from build123d import *

# Parameters (mm, degrees)
SKETCH1_W                = 114.3
SKETCH1_H                = 101.6
BOSS_EXTRUDE1_DEPTH      = 3.175
SKETCH2_W                = 114.3
SKETCH2_H                = 25.4
SKETCH2_H_2              = 19.05
BOSS_EXTRUDE2_DEPTH      = 3.175
M3_CLEARANCE_HOLE1_D     = 3.4
M3_CLEARANCE_HOLE1_DEPTH = 6.35
M3_CLEARANCE_HOLE1_TIP   = 1.021463052


with BuildPart() as part:
    # Sketch1 → Boss-Extrude1 (new body)
    with BuildSketch(Plane(origin=(0, 0, 0), x_dir=(1, 0, 0), z_dir=(0, 1, 0))):
        Rectangle(SKETCH1_W, SKETCH1_H)
    extrude(amount=BOSS_EXTRUDE1_DEPTH)

    # Sketch2 → Boss-Extrude2 (add)
    # profile 1 of 4: a face of its own
    with BuildSketch(Plane(origin=(0, 3.175, 0), x_dir=(1, 0, 0), z_dir=(0, 1, 0))):
        with BuildLine():
            Line((-76.2, -50.8), (-57.15, -50.8))
            Line((-57.15, -50.8), (-57.15, 50.8))
            Line((-57.15, 50.8), (-76.2, 50.8))
            Line((-76.2, 50.8), (-76.2, -25.4))
            ThreePointArc((-76.2, -25.4), (-88.9, -38.1), (-76.2, -50.8))
        make_face()
        with BuildLine():
            ThreePointArc((-76.2, -34.1), (-72.2, -38.1), (-76.2, -42.1))
            ThreePointArc((-76.2, -42.1), (-80.2, -38.1), (-76.2, -34.1))
        make_face(mode=Mode.SUBTRACT)
    # profile 2 of 4: a face of its own
    with BuildSketch(Plane(origin=(0, 3.175, 0), x_dir=(1, 0, 0), z_dir=(0, 1, 0))):
        with Locations((0, -63.5)):
            Rectangle(SKETCH2_W, SKETCH2_H)
    # profile 3 of 4: a face of its own
    with BuildSketch(Plane(origin=(0, 3.175, 0), x_dir=(1, 0, 0), z_dir=(0, 1, 0))):
        with BuildLine():
            Line((57.15, -50.8), (76.2, -50.8))
            ThreePointArc((76.2, -50.8), (88.9, -38.1), (76.2, -25.4))
            Line((76.2, -25.4), (76.2, 50.8))
            Line((76.2, 50.8), (57.15, 50.8))
            Line((57.15, 50.8), (57.15, -50.8))
        make_face()
        with BuildLine():
            ThreePointArc((76.2, -42.1), (72.2, -38.1), (76.2, -34.1))
            ThreePointArc((76.2, -34.1), (80.2, -38.1), (76.2, -42.1))
        make_face(mode=Mode.SUBTRACT)
    # profile 4 of 4: a face of its own
    with BuildSketch(Plane(origin=(0, 3.175, 0), x_dir=(1, 0, 0), z_dir=(0, 1, 0))):
        with Locations((0, 60.325)):
            Rectangle(SKETCH2_W, SKETCH2_H_2)
    extrude(amount=-BOSS_EXTRUDE2_DEPTH)

    # M3 Clearance Hole1
    with Locations(Plane(origin=(0, 3.175, 0), x_dir=(1, 0, 0), z_dir=(0, 1, 0))):
        with Locations((-76.2, -29.6), (-76.2, -46.6), (76.2, -29.6), (76.2, -46.6)):
            Hole(M3_CLEARANCE_HOLE1_D / 2, depth=M3_CLEARANCE_HOLE1_DEPTH)
            with Locations((0, 0, -(M3_CLEARANCE_HOLE1_DEPTH + M3_CLEARANCE_HOLE1_TIP / 2))):  # 118° drill point
                Cone(0, M3_CLEARANCE_HOLE1_D / 2, M3_CLEARANCE_HOLE1_TIP, mode=Mode.SUBTRACT)


solid = part.part
Check sheet for the modelled part. Datum: model origin and axes. Units: mm. Give positions to 0.01 mm unless a question says otherwise; leave off trailing zeros. Loops run counter-clockwise (first coordinate to the right, second up) from the corner with the lowest first, then second, coordinate; pieces in that order, holes last. Notation, with made-up numbers: M 24.5,3 L 28.5,3 A28 cw 28.5,34 Z; hole C 5.5,45.5 d9. An arc over 180 degrees is marked long. Return JSON: item names as keys, results as strings. Group by question number.
1. Go/stop test with flat-tipped pins: pin 1 (1.6 mm diameter, centred on y = 1.5, z = -12.5, fed in from -X); pin 2 (1 mm diameter, centred on x = 69.5, y = 2, fed in from +Z); pin 3 (1.5 mm diameter, centred on y = 2.5, z = -24.5, fed in from +X). Record where each tip stops, or that it passes through.
2. Thickness scan on L1, parallel to X at y = 1.05, z = 38.1; L2, parallel to X at y = 3, z = 35; L3, parallel to X at y = 2.15, z = 52. Record the ranges inside material, lowest first.
3. Cross-section at A-A on z = 38.1. Record the boundary of the cut face in (x, y) (3 decimals).
4. Cross-section at B-B on y = 0.6. Record the boundary of the cut face in (x, z).
5. Cross-section at D-D on z = 56.5. Record the boundary of the cut face in (x, y) (3 decimals).
6. Mould release check, pull along Z, two halves, no side actions. Record for faces 1 (the cylindrical face through (-88.897, 1.61, 37.821)), 2 (the cylindrical face through (-73.8, 1.6, 34.9)), 3 (the flat face through (-1, 3.175, 2)), 4 (the cylindrical face through (72.651, 1.61, 36.254)): released by +Z, released by -Z, zero draft, split by the parting line, or undercut.
7. Cross-section at C-C on z = -19.5. Record the boundary of the cut face in (x, y) (3 decimals).
Return value:
{
 "1": {"pin 1": "x = -76.2", "pin 2": "z = 50.8", "pin 3": "x = 76.2"},
 "2": {"L1": "-88.9 to -80.2, -72.2 to 72.2, 80.2 to 88.9", "L2": "-88.52 to -78.73, -73.67 to 73.67, 78.73 to 88.52", "L3": "-57.15 to 57.15"},
 "3": {"outline": "M -88.9,0 L -80.2,0 L -80.2,3.175 L -88.9,3.175 Z; M -72.2,0 L 72.2,0 L 72.2,3.175 L -72.2,3.175 Z; M 80.2,0 L 88.9,0 L 88.9,3.175 L 80.2,3.175 Z"},
 "4": {"outline": "M -76.2,-50.8 L -57.15,-50.8 L -57.15,-69.85 L 57.15,-69.85 L 57.15,-50.8 L 76.2,-50.8 L 76.2,25.4 A12.7 ccw 76.2,50.8 L 57.15,50.8 L 57.15,76.2 L -57.15,76.2 L -57.15,50.8 L -76.2,50.8 A12.7 ccw -76.2,25.4 Z; hole C -76.2,38.1 d8; hole C -76.2,29.6 d3.4; hole C -76.2,46.6 d3.4; hole C 76.2,38.1 d8; hole C 76.2,29.6 d3.4; hole C 76.2,46.6 d3.4"},
 "5": {"outline": "M -57.15,0 L 57.15,0 L 57.15,3.175 L -57.15,3.175 Z"},
 "6": {"face 1": "split by the parting line", "face 2": "undercut", "face 3": "zero draft", "face 4": "undercut"},
 "7": {"outline": "M -76.2,0 L 76.2,0 L 76.2,3.175 L -76.2,3.175 Z"}
}
